Design review of the part built by this model. Coordinates are the model's own, in mm. A direction names the side the tool comes from. Coordinates: 2 decimals unless noted, no trailing zeros. Write each loop counter-clockwise with the first axis right and the second up, starting at its lowest first coordinate (ties: lowest second). Pieces come first, ordered by that corner, then holes. Notation, with made-up numbers: (61, -26.75) - (94, -26.75) arc R36 ccw to (94, 10.25) - close; hole circle Ø9 at (23, 27). An arc over 180 degrees is marked (long way). Use a Markdown table: item, result.
Autodesk Inventor part; units mm, degrees
ref_plane "YZ Plane" through (0, 0, 0) normal (1, 0, 0) x (0, 1, 0)
ref_plane "XZ Plane" through (0, 0, 0) normal (0, 1, 0) x (-1, 0, 0)
ref_plane "XY Plane" through (0, 0, 0) normal (0, 0, 1) x (1, 0, 0)
sketch "Sketch1" plane through (0, 0, 0) normal (0, 0, 1) x (1, 0, 0)
  line L0 (-23.6135, 32.149) -> (26.3865, 32.149)
  line L1 (26.3865, 32.149) -> (26.3865, -17.851)
  line L2 (26.3865, -17.851) -> (-23.6135, -17.851)
  line L3 (-23.6135, -17.851) -> (-23.6135, 32.149)
  point P0 (0, 0)
  dimension "d0" = 50
  dimension "d1" = 50
extrude "Extrusion1" add sketch "Sketch1" along normal blind 30
sketch "Sketch2" plane through (0, 0, 30) normal (0, 0, 1) x (1, 0, 0)
  line L0 (12.3865, 22.149) -> (21.3865, 22.149)
  line L1 (21.3865, 22.149) -> (21.3865, -7.851)
  line L2 (21.3865, -7.851) -> (12.3865, -7.851)
  line L3 (12.3865, -7.851) -> (12.3865, 22.149)
  line L4 (-18.6135, 22.149) -> (-9.6135, 22.149)
  line L5 (-9.6135, 22.149) -> (-9.6135, -7.851)
  line L6 (-9.6135, -7.851) -> (-18.6135, -7.851)
  line L7 (-18.6135, -7.851) -> (-18.6135, 22.149)
  line L8 (26.3865, 32.149) -> (-23.6135, 32.149)
  line L9 (-23.6135, -17.851) -> (26.3865, -17.851)
  line L10 (26.3865, -17.851) -> (26.3865, 32.149)
  line L11 (-23.6135, 32.149) -> (-23.6135, -17.851)
  point P0 (0, 0)
  dimension "d4" = 10
  dimension "d5" = 10
  dimension "d6" = 5
  dimension "d7" = 5
  dimension "d11" = 9
  dimension "d12" = 9
sketch "Sketch3" plane through (-23.6135, -17.851, 0) normal (0, -1, 0) x (1, 0, 0)
  line L0 (0, 30) -> (50, 30)
  circle A0 centre (25, 30) radius 6
  point P0 (23.6135, 0)
  dimension "d8" = 12
  dimension "d13" = 25
extrude "Extrusion2" cut sketch "Sketch3" against normal blind 50
extrude "Extrusion3" add sketch "Sketch2" along normal blind 19 contours L0 L1 L2 L3 | L4 L5 L6 L7
equation "\"d1\" = d0"
properties part number "laser top" material "Iron, Cast"
(1) Take a section at B-B on x = -13.5. Write out the cut boundary in (y, z).
Determined:
| item | result |
|---|---|
| outline | (-17.85, 0) - (32.15, 0) - (32.15, 30) - (22.15, 30) - (22.15, 49) - (-7.85, 49) - (-7.85, 30) - (-17.85, 30) - close |
(2) Draft analysis for pull direction X (two halves, no side actions). For faces 1 (the flat face through (17, 7, 49)), 2 (the flat face through (21.386, 7, 39)), 3 (the flat face through (-23.614, 7, 15)), 4 (the cylindrical face through (1.3, 6.8, 24)), state which applies: +X half, -X half, draft (parallel to the pull), parting line (faces both ways), or undercut.
Determined:
| item | result |
|---|---|
| face 1 | draft |
| face 2 | +X half |
| face 3 | -X half |
| face 4 | undercut |
(3) Take a section at C-C on y = 3.5. Write out the cut boundary in (x, z), and give its area (3 significant figures).
Determined:
| item | result |
|---|---|
| outline | (-23.61, 0) - (26.39, 0) - (26.39, 30) - (21.39, 30) - (21.39, 49) - (12.39, 49) - (12.39, 30) - (7.39, 30) arc R6 cw to (-4.61, 30) - (-9.61, 30) - (-9.61, 49) - (-18.61, 49) - (-18.61, 30) - (-23.61, 30) - close |
| area | 1,790 mm2 |
(4) Take a section at A-A on z = 33. Write out the cut boundary in (x, y), and give its area (3 significant figures).
Determined:
| item | result |
|---|---|
| outline | (-18.61, -7.85) - (-9.61, -7.85) - (-9.61, 22.15) - (-18.61, 22.15) - close; (12.39, -7.85) - (21.39, -7.85) - (21.39, 22.15) - (12.39, 22.15) - close |
| area | 540 mm2 |
(5) For L1, parallel to X at y = 21, z = 39; L2, parallel to Z at x = 1.5, y = -1; L3, parallel to Z at x = -13.5, y = -9.5, list the stretches that pass through material, from the lowest coordinate up. Write a range as from..to.
Determined:
| item | result |
|---|---|
| L1 | -18.61..-9.61, 12.39..21.39 |
| L2 | 0..24 |
| L3 | 0..30 |
(6) For pin 1 (7 mm diameter, centred on x = 15, z = 37.5, fed in from -Y); pin 2 (10 mm diameter, centred on x = 16.5, z = 40.5, fed in from +Y); pin 3 (9.5 mm diameter, centred on y = 1, z = 39, fed in from -X), all flat-tipped, find the tip position at first contact; note any pin that passes through.
Determined:
| item | result |
|---|---|
| pin 1 | y = -7.85 |
| pin 2 | y = 22.15 |
| pin 3 | x = -18.61 |
(7) Take a section at D-D on y = 27. Write out the cut boundary in (x, z), and give its area (3 significant figures).
Determined:
| item | result |
|---|---|
| outline | (-23.61, 0) - (26.39, 0) - (26.39, 30) - (7.39, 30) arc R6 cw to (-4.61, 30) - (-23.61, 30) - close |
| area | 1,440 mm2 |
(8) Machinability: for faces 5 (the flat face through (17, 22.149, 39)), 6 (the flat face through (1, 7, 0)), 7 (the flat face through (12.386, 7, 39)), 8 (the flat face through (-14, -7.851, 39)), 9 (the flat face through (-18.614, 7, 39)), which of the approach directions +Z, -Z, +X, -X, +Y, -Y give a long, thin tool a straight path to every point of the face, cutting with its end or side? Answer none if there is none.
Determined:
| item | result |
|---|---|
| face 5 | +Z, +X, -X, +Y |
| face 6 | -Z, +X, -X, +Y, -Y |
| face 7 | +Z, +Y, -Y |
| face 8 | +Z, +X, -X, -Y |
| face 9 | +Z, -X, +Y, -Y |
